```python
from build123d import *

# Parameters (mm, degrees)
CHAMFER_1_SIZE         = 1
CHAMFER_1_SIZE2        = 0.577350269
CHAMFER_1_PART_2_SIZE  = 1
CHAMFER_1_PART_2_SIZE2 = 0.577350269
CUT_EXTRUDE_1_DEPTH    = 5
CUT_EXTRUDE_2_DEPTH    = 5


with BuildPart() as part:
    # Эскиз1 → Повернуть1 (revolve)
    with BuildSketch(Plane(origin=(0, 0, 0), x_dir=(0, 0, -1), z_dir=(1, 0, 0))):
        Polygon((0, 17.25), (0, 60), (4, 60), (4, 25), (20, 25), (20, 18), (16, 18), (16, 22.5), (8, 22.5), (8, 17.25), align=None)
    revolve(axis=Axis((0, 0, 0), (0, 0, -1)))

    # Фаска1
    chamfer_1_edges = [part.edges().sort_by_distance(p)[0] for p in [
        (0, -17.25, 0),
    ]]
    chamfer_1_side = [part.faces().sort_by_distance(p)[0] for p in [
        (0, -18.947056275, 0),
    ]]
    chamfer(chamfer_1_edges, length=CHAMFER_1_SIZE, length2=CHAMFER_1_SIZE2, reference=chamfer_1_side[0])

    # Фаска1 part 2
    chamfer_1_part_2_edges = [part.edges().sort_by_distance(p)[0] for p in [
        (0, -17.25, -8),
    ]]
    chamfer_1_part_2_side = [part.faces().sort_by_distance(p)[0] for p in [
        (0, -21.863603897, -8),
    ]]
    chamfer(chamfer_1_part_2_edges, length=CHAMFER_1_PART_2_SIZE, length2=CHAMFER_1_PART_2_SIZE2, reference=chamfer_1_part_2_side[0])

    # Эскиз2 → Вырез-Вытянуть1 (cut)
    with BuildSketch(Plane(origin=(0, 0, -20), x_dir=(-1, 0, 0), z_dir=(0, 0, -1))):
        with BuildLine():
            ThreePointArc((17, 18.33030278), (0, 25), (-17, 18.33030278))
            Line((-17, 18.33030278), (-17, 5.916079783))
            ThreePointArc((-17, 5.916079783), (0, 18), (17, 5.916079783))
            Line((17, 5.916079783), (17, 18.33030278))
        make_face()
        with BuildLine():
            Line((-17, -5.916079783), (-17, -18.33030278))
            ThreePointArc((-17, -18.33030278), (0, -25), (17, -18.33030278))
            Line((17, -18.33030278), (17, -5.916079783))
            ThreePointArc((17, -5.916079783), (0, -18), (-17, -5.916079783))
        make_face()
    extrude(amount=-CUT_EXTRUDE_1_DEPTH, mode=Mode.SUBTRACT)

    # Эскиз3 → Вырез-Вытянуть2 (cut)
    with BuildSketch(Plane.XY):
        with BuildLine():
            Line((-9, 23.323807579), (-9, 59.3211598))
            ThreePointArc((-9, 59.3211598), (-39.115214431, -45.497252664), (60, 0))
            ThreePointArc((60, 0), (45.497252664, 39.115214431), (9, 59.3211598))
            Line((9, 59.3211598), (9, 23.323807579))
            ThreePointArc((9, 23.323807579), (20.615528128, 14.142135624), (25, 0))
            ThreePointArc((25, 0), (-14.142135624, -20.615528128), (-9, 23.323807579))
        make_face()
    extrude(amount=-CUT_EXTRUDE_2_DEPTH, mode=Mode.SUBTRACT)


solid = part.part
```
Verification items for the finished model (mm, model axes). A direction names the side the tool comes from. Round coordinates to 2 decimals unless told otherwise and drop trailing zeros. Write each loop counter-clockwise with the first axis right and the second up, starting at its lowest first coordinate (ties: lowest second). Pieces come first, ordered by that corner, then holes. Notation, with made-up numbers: (52.25, 4.5) - (90.25, 4.5) arc R14 cw to (90.25, 31.5) - close; hole circle Ø11 at (19.25, -39.75). An arc over 180 degrees is marked (long way). Answer as a JSON object with one key per item and string values. Group by question number.
Q1. Section check C-C, the plane z = -3. Enter the section's corners in (x, y).
Q2. Mould release check, pull along Y, two halves, no side actions. Record for faces 6 (the flat face through (-19, 0, -16)), 7 (the cylindrical face through (-15, -20, -10)), 8 (the flat face through (0, 23, -15)): released by +Y, released by -Y, zero draft, split by the parting line, or undercut.
Q3. Section check B-B, the plane y = 0. Enter the section's corners in (x, z).
Q4. Go/stop test with flat-tipped pins: pin 1 Ø5 at (x, y) = (0, -21) entering from -Z; pin 2 Ø2.5 at (y, z) = (-10, -17) entering from +X; pin 3 Ø13.5 at (x, y) = (4, 10.5) entering from -Z. Record where each tip stops, or that it passes through.
Q5. Thickness scan on line 1 (Y direction, x = 0, z = -13.25); line 2 (Z direction, x = -5.5, y = 30). Record the ranges inside material, lowest first.
Q6. Tool access check on faces 1 (the cylindrical face through (18, 0, -18)), 2 (the cylindrical face through (5.181, 16.453, -3.952)), 3 (the flat face through (-9, 41, -2)), 4 (the flat face through (-17, 12, -18)), 5 (the flat face through (19, 0, -16)). Record the directions out of +Z, -Z, +X, -X, +Y, -Y that give a thin tool (end or side, any length) a straight path to the whole face; none if there is none.
Q7. Section check A-A, the plane x = 0. Enter the section's corners in (y, z), plus the area to 3 significant figures.
Q8. Section check D-D, the plane z = -9. Enter the section's corners in (x, y), plus the area to 3 significant figures.
Found:
{
 "1": {"outline": "(-9, 23.32) arc R25 ccw (long way) to (9, 23.32) - (9, 59.32) arc R60 ccw to (-9, 59.32) - close; hole circle Ø34.5 at (0, 0)"},
 "2": {"face 6": "undercut", "face 7": "split by the parting line", "face 8": "zero draft"},
 "3": {"outline": "(-25, -20) - (-18, -20) - (-18, -16) - (-22.5, -16) - (-22.5, -8) - (-18.25, -8) - (-17.25, -7.42) - (-17.25, -0.58) - (-18.25, 0) - (-25, 0) - close; (17.25, -7.42) - (18.25, -8) - (22.5, -8) - (22.5, -16) - (18, -16) - (18, -20) - (25, -20) - (25, 0) - (18.25, 0) - (17.25, -0.58) - close"},
 "4": {"pin 1": "stops at z = -15", "pin 2": "stops at x = 23.42", "pin 3": "stops at z = -7.85"},
 "5": {"line 1": "y = -25 to -22.5, 22.5 to 25", "line 2": "z = -4 to 0"},
 "6": {"face 1": "-Z", "face 2": "+Z, -Z", "face 3": "+Z, -Z, -X, +Y", "face 4": "-Z, +Y, -Y", "face 5": "none"},
 "7": {"outline": "(-25, -15) - (-22.5, -15) - (-22.5, -8) - (-18.25, -8) - (-17.25, -7.42) - (-17.25, -0.58) - (-18.25, 0) - (-25, 0) - close; (17.25, -7.42) - (18.25, -8) - (22.5, -8) - (22.5, -15) - (25, -15) - (25, -4) - (60, -4) - (60, 0) - (18.25, 0) - (17.25, -0.58) - close", "area": "298 mm^2"},
 "8": {"outline": "circle Ø50 at (0, 0); hole circle Ø45 at (0, 0)", "area": "373 mm^2"}
}
